```python
from build123d import *

# Parameters (mm, degrees)
BOSS_EXTRUDE1_DEPTH = 4
CUT_EXTRUDE1_DEPTH  = 94.973453698
SKETCH5_W           = 4
SKETCH5_H           = 19.8
BOSS_EXTRUDE2_DEPTH = 4
CUT_EXTRUDE2_DEPTH  = 96.321613499


with BuildPart() as part:
    # Sketch1 → Boss-Extrude1 (new body)
    with BuildSketch(Plane.XY):
        Polygon((-9.9, 85), (-9.9, 89), (9.9, 89), (9.9, 85), (29.9, 85), (29.9, -85), (-29.9, -85), (-29.9, 85), align=None)
    extrude(amount=BOSS_EXTRUDE1_DEPTH)

    # Sketch3 → Cut-Extrude1 (cut, through all)
    with BuildSketch(Plane(origin=(0, 0, 0), x_dir=(-1, 0, 0), z_dir=(0, 0, -1))):
        Polygon((23, 85), (23, 80.9), (21.5, 80.9), (21.5, 76.9), (22.9, 76.9), (22.9, 73.9), (21.5, 73.9), (21.5, 70), (18.3, 70), (18.3, 73.9), (16.9, 73.9), (16.9, 76.9), (18.3, 76.9), (18.3, 80.9), (16.8, 80.9), (16.8, 85), align=None)
        Polygon((-16.8, 85), (-16.8, 80.9), (-18.3, 80.9), (-18.3, 76.9), (-16.9, 76.9), (-16.9, 73.9), (-18.3, 73.9), (-18.3, 70), (-21.5, 70), (-21.5, 73.9), (-22.9, 73.9), (-22.9, 76.9), (-21.5, 76.9), (-21.5, 80.9), (-23, 80.9), (-23, 85), align=None)
        Polygon((-23, -85), (-23, -80.9), (-21.5, -80.9), (-21.5, -76.9), (-22.9, -76.9), (-22.9, -73.9), (-21.5, -73.9), (-21.5, -70), (-18.3, -70), (-18.3, -73.9), (-16.9, -73.9), (-16.9, -76.9), (-18.3, -76.9), (-18.3, -80.9), (-16.8, -80.9), (-16.8, -85), align=None)
        Polygon((16.8, -85), (16.8, -80.9), (18.3, -80.9), (18.3, -76.9), (16.9, -76.9), (16.9, -73.9), (18.3, -73.9), (18.3, -70), (21.5, -70), (21.5, -73.9), (22.9, -73.9), (22.9, -76.9), (21.5, -76.9), (21.5, -80.9), (23, -80.9), (23, -85), align=None)
    extrude(amount=-CUT_EXTRUDE1_DEPTH, mode=Mode.SUBTRACT)

    # Sketch5 → Boss-Extrude2 (add)
    with BuildSketch(Plane.XY.offset(4)):
        with Locations((-31.9, 55.1)):
            Rectangle(SKETCH5_W, SKETCH5_H)
        with Locations((-31.9, 15.1)):
            Rectangle(SKETCH5_W, SKETCH5_H)
        with Locations((-31.9, -24.9)):
            Rectangle(SKETCH5_W, SKETCH5_H)
        with Locations((-31.9, -64.9)):
            Rectangle(SKETCH5_W, SKETCH5_H)
    extrude(amount=-BOSS_EXTRUDE2_DEPTH)

    # Sketch6 → Cut-Extrude2 (cut, through all)
    with BuildSketch(Plane.XY.offset(4)):
        with BuildLine():
            Line((-5, 30), (5, 30))
            ThreePointArc((5, 30), (12.071067812, 27.071067812), (15, 20))
            Line((15, 20), (15, -20))
            ThreePointArc((15, -20), (12.071067812, -27.071067812), (5, -30))
            Line((5, -30), (-5, -30))
            ThreePointArc((-5, -30), (-12.071067812, -27.071067812), (-15, -20))
            Line((-15, -20), (-15, 20))
            ThreePointArc((-15, 20), (-12.071067812, 27.071067812), (-5, 30))
        make_face()
    extrude(amount=-CUT_EXTRUDE2_DEPTH, mode=Mode.SUBTRACT)


solid = part.part
```
The model under review builds one solid part; all positions refer to its coordinate system, in mm. A direction names the side the tool comes from. Coordinates: 2 decimals unless noted, no trailing zeros. Write each loop counter-clockwise with the first axis right and the second up, starting at its lowest first coordinate (ties: lowest second). Pieces come first, ordered by that corner, then holes.
1) We need section B-B on y = 13. State the section outline as (x, z) points.
2) We need section A-A on x = -1.5. State the section outline as (y, z) points, then the cut area to 3 significant figures.
3) We need section D-D on y = -39. State the section outline as (x, z) points.
4) Machinability: for faces 5 (the face through (-18.3, 72, 2)), 6 (the face through (-22.9, 75, 2)), 7 (the face through (-32, -34.8, 2)), which of the approach directions +Z, -Z, +X, -X, +Y, -Y give a long, thin tool a straight path to every point of the face, cutting with its end or side? Answer none if there is none.
5) We need section C-C on x = -25.5. State the section outline as (y, z) points, then the cut area to 3 significant figures.
6) The part is to be moulded in two halves that separate along Y. For faces 1 (the face through (-16.8, -83, 2)), 2 (the face through (-32, -15, 2)), 3 (the face through (-20, -70, 2)), 4 (the face through (-29.9, 35, 2)), say which applies: pulls with the +Y half, pulls with the -Y half, needs draft (parallel to the pull), parting line crosses it, or undercut.
7) Clearance check with flat-ended pins moving along their axes: pin 1 Ø2 at (y, z) = (-5, 1.5) entering from -X; pin 2 Ø3 at (x, y) = (-22.5, 45.5) entering from -Z; pin 3 Ø0.8 at (x, z) = (-18, 3) entering from +Y; pin 4 Ø0.7 at (x, z) = (18, 2.5) entering from -Y. State where each tip first meets the part, or that it passes through.
8) To check wall thickness, follow probe 1 along X at (y, z) = (74.5, 1.6); probe 2 along X at (y, z) = (-77.5, 1.25); probe 3 along X at (y, z) = (-3, 2.5). State the ranges of each line that lie inside material, in increasing order.
Answer list:
1. outline: (-33.9, 0) - (-15, 0) - (-15, 4) - (-33.9, 4) - close; (15, 0) - (29.9, 0) - (29.9, 4) - (15, 4) - close
2. outline: (-85, 0) - (-30, 0) - (-30, 4) - (-85, 4) - close; (30, 0) - (89, 0) - (89, 4) - (30, 4) - close
2. area: 456 mm2
3. outline: (-29.9, 0) - (29.9, 0) - (29.9, 4) - (-29.9, 4) - close
4. face 5: +Z, -Z, +Y
4. face 6: +Z, -Z
4. face 7: +Z, -Z, -X
5. outline: (-85, 0) - (85, 0) - (85, 4) - (-85, 4) - close
5. area: 680 mm2
6. face 1: needs draft
6. face 2: undercut
6. face 3: pulls with the -Y half
6. face 4: undercut
7. pin 1: stops at x = -29.9
7. pin 2: stops at z = 0
7. pin 3: stops at y = 80.9
7. pin 4: stops at y = -80.9
8. probe 1: x = -29.9 to -22.9, -16.9 to 16.9, 22.9 to 29.9
8. probe 2: x = -29.9 to -21.5, -18.3 to 18.3, 21.5 to 29.9
8. probe 3: x = -29.9 to -15, 15 to 29.9
